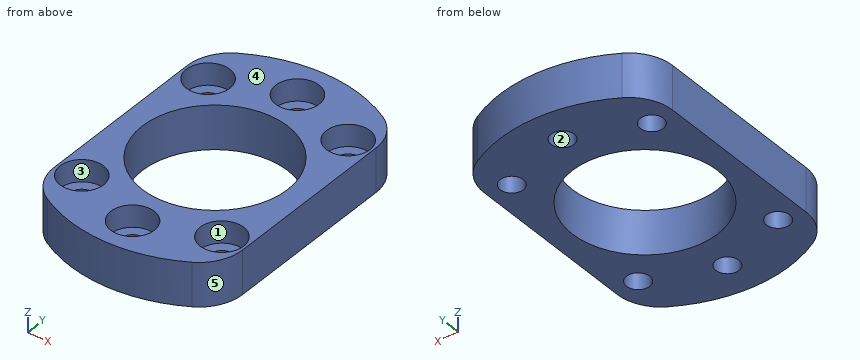
from build123d import *

# Parameters (mm, degrees)
SKETCH_1_R          = 10
EXTRUDE_1_DEPTH     = 6
SKETCH_2_R          = 1.6
CUT_EXTRUDE_1_DEPTH = 7
FILLET_1_R          = 6
FILLET_2_R          = 6
FILLET_3_R          = 6
FILLET_4_R          = 6
SKETCH_3_R          = 3
CUT_EXTRUDE_2_DEPTH = 3


with BuildPart() as part:
    # 草图1 → 拉伸1 (new body)
    with BuildSketch(Plane.XY):
        with BuildLine():
            Line((-12.98, 15.202621484), (-12.98, -15.202621484))
            ThreePointArc((-12.98, -15.202621484), (0, -19.99), (12.98, -15.202621484))
            Line((12.98, -15.202621484), (12.98, 15.202621484))
            ThreePointArc((12.98, 15.202621484), (0, 19.99), (-12.98, 15.202621484))
        make_face()
        Circle(SKETCH_1_R, mode=Mode.SUBTRACT)
    extrude(amount=EXTRUDE_1_DEPTH)

    # 草图2 → 切除-拉伸1 (cut)
    with BuildSketch(Plane.XY.offset(6)):
        with Locations((-9.641814145, 11.490666647)):
            Circle(SKETCH_2_R)
        with Locations((0, 15)):
            Circle(SKETCH_2_R)
        with Locations((9.641814145, 11.490666647)):
            Circle(SKETCH_2_R)
        with Locations((-9.641814145, -11.490666647)):
            Circle(SKETCH_2_R)
        with Locations((0, -15)):
            Circle(SKETCH_2_R)
        with Locations((9.641814145, -11.490666647)):
            Circle(SKETCH_2_R)
    extrude(amount=-CUT_EXTRUDE_1_DEPTH, mode=Mode.SUBTRACT)

    # 圆角1
    fillet_1_edges = [part.edges().sort_by_distance(p)[0] for p in [
        (-12.98, 15.202621484, 3),
    ]]
    fillet(fillet_1_edges, radius=FILLET_1_R)

    # 圆角2
    fillet_2_edges = [part.edges().sort_by_distance(p)[0] for p in [
        (12.98, 15.202621484, 3),
    ]]
    fillet(fillet_2_edges, radius=FILLET_2_R)

    # 圆角3
    fillet_3_edges = [part.edges().sort_by_distance(p)[0] for p in [
        (-12.98, -15.202621484, 3),
    ]]
    fillet(fillet_3_edges, radius=FILLET_3_R)

    # 圆角4
    fillet_4_edges = [part.edges().sort_by_distance(p)[0] for p in [
        (12.98, -15.202621484, 3),
    ]]
    fillet(fillet_4_edges, radius=FILLET_4_R)

    # 草图3 → 切除-拉伸2 (cut)
    with BuildSketch(Plane.XY.offset(6)):
        with Locations((-9.641814145, 11.490666647)):
            Circle(SKETCH_3_R)
        with Locations((0, 15)):
            Circle(SKETCH_3_R)
        with Locations((9.641814145, 11.490666647)):
            Circle(SKETCH_3_R)
        with Locations((-9.641814145, -11.490666647)):
            Circle(SKETCH_3_R)
        with Locations((0, -15)):
            Circle(SKETCH_3_R)
        with Locations((9.641814145, -11.490666647)):
            Circle(SKETCH_3_R)
    extrude(amount=-CUT_EXTRUDE_2_DEPTH, mode=Mode.SUBTRACT)


solid = part.part
Work out the finished part from the listing and answer in its coordinate system (mm). Face numbers are marked on the shaded views. A direction names the side the tool comes from. Coordinates: 2 decimals unless noted, no trailing zeros. Loops run counter-clockwise (first coordinate to the right, second up) from the corner with the lowest first, then second, coordinate; pieces in that order, holes last. Notation, with made-up numbers: M 20,-16 L 39,-16 A25 cw 39,-1 Z; hole C 89.5,8 d8. An arc over 180 degrees is marked long. Answer in a Markdown table with one row per item. Add a question column.
1. A tool of negligible diameter and unlimited length cuts with its end or side. For the marked faces 1 and 2, from which of +Z, -Z, +X, -X, +Y, -Y can it reach the whole face along a straight path? Write none if from no direction.
2. Flat-ended cylindrical pins translate along their axes: P1, Ø3.5, axis at x = 9.64, y = 11.49, coming from the +Z side; P2, Ø1.9, axis at x = 0, y = 15, coming from the -Z side. Find the tip coordinate at first contact, or state that the pin passes through.
3. Find section B-B, the plane x = 0. Write down the section's boundary in (y, z), then the cut area to 3 significant figures.
4. Consider L1, parallel to Y at x = 0, z = 0.6; L2, parallel to X at y = 11.5, z = 2.6; L3, parallel to Y at x = -10.75, z = 4.65. Determine where each line is inside the solid, lowest interval first.
5. The mould has two halves that part along X. Classify the marked faces 3, 4 and 5: pulls with the +X half, pulls with the -X half, needs draft (parallel to the pull), parting line crosses it, or undercut.
6. Find section D-D, the plane y = 0. Write down the section's boundary in (x, z), then the cut area to 3 significant figures.
7. Find section A-A, the plane y = -6. Write down the section's boundary in (x, z).
8. Find section C-C, the plane z = 5.2. Write down the section's boundary in (x, y), then the cut area to 3 significant figures.
Reported:
| question | item | result |
|---|---|---|
| 1 | face 1 | +Z |
| 1 | face 2 | +Z, -Z |
| 2 | P1 | stops at z = 3 |
| 2 | P2 | passes through |
| 3 | outline | M -19.99,0 L -16.6,0 L -16.6,3 L -18,3 L -18,6 L -19.99,6 Z; M -13.4,0 L -10,0 L -10,6 L -12,6 L -12,3 L -13.4,3 Z; M 10,0 L 13.4,0 L 13.4,3 L 12,3 L 12,6 L 10,6 Z; M 16.6,0 L 19.99,0 L 19.99,6 L 18,6 L 18,3 L 16.6,3 Z |
| 3 | area | 64.7 mm^2 |
| 4 | L1 | y = -19.99 to -16.6, -13.4 to -10, 10 to 13.4, 16.6 to 19.99 |
| 4 | L2 | x = -12.98 to -11.24, -8.04 to 8.04, 11.24 to 12.98 |
| 4 | L3 | y = -16.79 to -14.28, -8.7 to 8.7, 14.28 to 16.79 |
| 5 | face 3 | undercut |
| 5 | face 4 | needs draft |
| 5 | face 5 | pulls with the +X half |
| 6 | outline | M -12.98,0 L -10,0 L -10,6 L -12.98,6 Z; M 10,0 L 12.98,0 L 12.98,6 L 10,6 Z |
| 6 | area | 35.8 mm^2 |
| 7 | outline | M -12.98,0 L -8,0 L -8,6 L -12.98,6 Z; M 8,0 L 12.98,0 L 12.98,6 L 8,6 Z |
| 8 | outline | M -12.98,-12.12 A6 ccw -9.97,-17.32 A19.99 ccw 9.97,-17.32 A6 ccw 12.98,-12.12 L 12.98,12.12 A6 ccw 9.97,17.32 A19.99 ccw -9.97,17.32 A6 ccw -12.98,12.12 Z; hole C -9.64,-11.49 d6; hole C -9.64,11.49 d6; hole C 0,0 d20; hole C 0,-15 d6; hole C 0,15 d6; hole C 9.64,-11.49 d6; hole C 9.64,11.49 d6 |
| 8 | area | 469 mm^2 |
